The listing builds one solid part. Answer for the finished solid, in the listing's coordinates (mm). A direction names the side the tool comes from. Give positions to 0.01 mm unless a question says otherwise; leave off trailing zeros. Order: outer loops, then holes, each group sorted by start corner. A loop starts at its lowest first (then second) coordinate and runs counter-clockwise, first axis right, second up. Notation, with made-up numbers: (13.5, -17.75) - (47.5, -17.75) arc R9 ccw to (47.5, -2.75) - close; hole circle Ø5 at (-22, 0.5). An arc over 180 degrees is marked (long way). Write each question's results on one line, items separated by ' | '. Start each with the question number.
1. Section A-A (x = -12.01) is taken. Give the vertices of the cut face in (y, z), and give its area (3 significant figures).
2. Find the intervals of material crossed by L1, parallel to X at y = 18, z = -4 (3 decimals); L2, parallel to Y at x = -12.01, z = 2; L3, parallel to Y at x = 12.09, z = 2.25, in increasing order.
3. Section D-D (y = 3.8) is taken. Give the vertices of the cut face in (x, z).
4. Flat-ended cylindrical pins translate along their axes: pin 1 (2 mm diameter, centred on x = 9, z = -5.5, fed in from +Y); pin 2 (0.8 mm diameter, centred on x = -11.5, z = 6, fed in from -Y); pin 3 (6 mm diameter, centred on y = 15.5, z = 0.5, fed in from +X); pin 4 (3 mm diameter, centred on x = 11.5, y = 2, fed in from -Z). Find the tip coordinate at first contact, or state that the pin passes through.
5. Section B-B (z = 0) is taken. Give the vertices of the cut face in (x, y) (3 decimals), and give its area (3 significant figures).
6. Section C-C (x = 12.09) is taken. Give the vertices of the cut face in (y, z), and give its area (3 significant figures).
7. Determine the mould class of faces 1 (the face through (-8.464, 26.03, -0.134)), 2 (the face through (13.4, 18.4, -5.15)), 3 (the face through (13.4, 7.1, 0)), 4 (the face through (-12, 19.828, -6)) for opening direction Z: released by +Z, released by -Z, zero draft, split by the parting line, or undercut.
8. Which of the six approach directions +Z, -Z, +X, -X, +Y, -Y give full straight-line access (tool end or side, diameter ignored) to faces 5 (the face through (8.484, 26.03, 0.134)), 6 (the face through (12, 14.372, -6)), 7 (the face through (9.716, 15.755, 6.418)), 8 (the face through (11.48, 3.09, 5.38)), 9 (the face through (-13, 3, 0))?
from build123d import *

# Parameters (mm, degrees)
SKETCH1_W                    = 34.42
SKETCH1_H                    = 15.3
BOSS_EXTRUDE1_DEPTH          = 21.1
CHAMFER1_SIZE                = 3.6
CHAMFER1_SIZE2               = 2.7
CHAMFER2_SIZE                = 4.2
CHAMFER2_SIZE2               = 3.3
CUT_EXTRUDE1_DEPTH           = 32.232740834
SKETCH3_R                    = 8.475
BOSS_EXTRUDE2_DEPTH          = 10
CUT_EXTRUDE2_REACH           = 30.517
F_0_15_0_15_DIAMETER_HOLE1_D = 3.3
F_0_15_0_15_DIAMETER_HOLE2_D = 3.3
CUT_EXTRUDE3_DEPTH           = 2.5
CUT_EXTRUDE4_START           = -15.3
CUT_EXTRUDE4_DEPTH           = 2.5
SKETCH10_W                   = 6.1
SKETCH10_H                   = 6.1
CUT_EXTRUDE5_DEPTH           = 7.7
CUT_EXTRUDE6_DEPTH           = 7.7
SKETCH12_R                   = 3
BOSS_EXTRUDE3_DEPTH          = 13


with BuildPart() as part:
    # Sketch1 → Boss-Extrude1 (new body)
    with BuildSketch(Plane(origin=(0, 0, 0), x_dir=(1, 0, 0), z_dir=(0, 1, 0))):
        Rectangle(SKETCH1_W, SKETCH1_H)
    extrude(amount=BOSS_EXTRUDE1_DEPTH)

    # Chamfer1
    chamfer1_edges = [part.edges().sort_by_distance(p)[0] for p in [
        (17.21, 21.1, 0),
    ]]
    chamfer1_side = [part.faces().sort_by_distance(p)[0] for p in [
        (17.21, 10.55, 0),
    ]]
    chamfer(chamfer1_edges, length=CHAMFER1_SIZE, length2=CHAMFER1_SIZE2, reference=chamfer1_side[0])

    # Chamfer2
    chamfer2_edges = [part.edges().sort_by_distance(p)[0] for p in [
        (-17.21, 21.1, 0),
    ]]
    chamfer2_side = [part.faces().sort_by_distance(p)[0] for p in [
        (-17.21, 10.55, 0),
    ]]
    chamfer(chamfer2_edges, length=CHAMFER2_SIZE, length2=CHAMFER2_SIZE2, reference=chamfer2_side[0])

    # Sketch2 → Cut-Extrude1 (cut, through all)
    with BuildSketch(Plane.XY.offset(7.65)):
        Polygon((-17.21, 3), (-7.71, 3), (-6.91, 0), (-17.21, 0), align=None)
        Polygon((17.21, 6.1), (13.11, 6.1), (9.81, 0), (17.21, 0), align=None)
    extrude(amount=-CUT_EXTRUDE1_DEPTH, mode=Mode.SUBTRACT)

    # Sketch3 → Boss-Extrude2 (add)
    with BuildSketch(Plane(origin=(0, 21.1, 0), x_dir=(1, 0, 0), z_dir=(0, 1, 0))):
        with Locations(Location((0.01, 0, 0), (0, 0, 64.509262206))):
            Circle(SKETCH3_R)
    extrude(amount=BOSS_EXTRUDE2_DEPTH)

    # Sketch4 → Cut-Extrude2 (cut, up to next)
    with BuildSketch(Plane.XZ.offset(-21.1), mode=Mode.PRIVATE) as cut_extrude2_sk1:
        with BuildLine():
            Line((-3.637344925, -7.65), (3.657344925, -7.65))
            ThreePointArc((3.657344925, -7.65), (0.01, -8.475), (-3.637344925, -7.65))
        make_face()
    cut_extrude2_tool1 = extrude(cut_extrude2_sk1.sketch, amount=-CUT_EXTRUDE2_REACH, mode=Mode.PRIVATE) & part.part
    # Sketch4 → Cut-Extrude2 (cut, up to next)
    with BuildSketch(Plane.XZ.offset(-21.1), mode=Mode.PRIVATE) as cut_extrude2_sk2:
        with BuildLine():
            Line((-3.637344925, 7.65), (3.657344925, 7.65))
            ThreePointArc((3.657344925, 7.65), (0.01, 8.475), (-3.637344925, 7.65))
        make_face()
    cut_extrude2_tool2 = extrude(cut_extrude2_sk2.sketch, amount=-CUT_EXTRUDE2_REACH, mode=Mode.PRIVATE) & part.part
    add(cut_extrude2_tool1.solids().sort_by_distance((0.01, 21.1, -7.981417))[0], mode=Mode.SUBTRACT)
    add(cut_extrude2_tool2.solids().sort_by_distance((0.01, 21.1, 7.981417))[0], mode=Mode.SUBTRACT)

    # Ø0.15 (0.15) Diameter Hole1 (through all)
    with Locations(Plane.XY.offset(7.65)):
        with Locations((-12.01, 17.1)):
            Hole(F_0_15_0_15_DIAMETER_HOLE1_D / 2)

    # Ø0.15 (0.15) Diameter Hole2 (through all)
    with Locations(Plane.XY.offset(7.65)):
        with Locations((12.09, 17.1)):
            Hole(F_0_15_0_15_DIAMETER_HOLE2_D / 2)

    # Sketch9 → Cut-Extrude3 (cut)
    with BuildSketch(Plane.XY.offset(7.65)):
        Polygon((8.94, 17.1), (10.515, 14.372019978), (13.665, 14.372019978), (15.24, 17.1), (13.665, 19.827980022), (10.515, 19.827980022), align=None)
        Polygon((-15.16, 17.1), (-13.585, 14.372019978), (-10.435, 14.372019978), (-8.86, 17.1), (-10.435, 19.827980022), (-13.585, 19.827980022), align=None)
    extrude(amount=-CUT_EXTRUDE3_DEPTH, mode=Mode.SUBTRACT)

    # Sketch9<2> → Cut-Extrude4 (cut)
    with BuildSketch(Plane.XY.offset(7.65).offset(CUT_EXTRUDE4_START)):
        Polygon((8.94, 17.1), (10.515, 14.372019978), (13.665, 14.372019978), (15.24, 17.1), (13.665, 19.827980022), (10.515, 19.827980022), align=None)
        Polygon((-15.16, 17.1), (-13.585, 14.372019978), (-10.435, 14.372019978), (-8.86, 17.1), (-10.435, 19.827980022), (-13.585, 19.827980022), align=None)
    extrude(amount=CUT_EXTRUDE4_DEPTH, mode=Mode.SUBTRACT)

    # Sketch10 → Cut-Extrude5 (cut)
    with BuildSketch(Plane(origin=(17.21, 0, 0), x_dir=(0, 0, -1), z_dir=(1, 0, 0))):
        with Locations((0, 3.05)):
            Rectangle(SKETCH10_W, SKETCH10_H)
    extrude(amount=-CUT_EXTRUDE5_DEPTH, mode=Mode.SUBTRACT)

    # Sketch11 → Cut-Extrude6 (cut)
    with BuildSketch(Plane(origin=(17.21, 0, 0), x_dir=(0, 0, -1), z_dir=(1, 0, 0))):
        with BuildLine():
            Line((2, 6.1), (-2, 6.1))
            ThreePointArc((-2, 6.1), (0, 7.1), (2, 6.1))
        make_face()
    extrude(amount=-CUT_EXTRUDE6_DEPTH, mode=Mode.SUBTRACT)

    # Sketch12 → Boss-Extrude3 (add)
    with BuildSketch(Plane(origin=(9.51, 0, 0), x_dir=(0, 0, -1), z_dir=(1, 0, 0))):
        with Locations(Location((0, 3.8, 0), (0, 0, 180))):
            Circle(SKETCH12_R)
    extrude(amount=BOSS_EXTRUDE3_DEPTH)


solid = part.part
Reported:
1) outline: (3, -7.65) - (14.37, -7.65) - (14.37, -5.15) - (15.45, -5.15) - (15.45, 5.15) - (14.37, 5.15) - (14.37, 7.65) - (3, 7.65) - close; (18.75, -5.15) - (19.83, -5.15) - (19.83, -7.65) - (21.1, -7.65) - (21.1, 7.65) - (19.83, 7.65) - (19.83, 5.15) - (18.75, 5.15) - close | area: 216 mm²
2) L1: -16.346 to -13.393, -10.627 to 10.707, 13.473 to 16.835 | L2: 3 to 15.45, 18.75 to 21.1 | L3: 1.82 to 5.78, 6.1 to 15.45, 18.75 to 21.1
3) outline: (-17.21, -7.65) - (11.87, -7.65) - (11.87, -3.05) - (9.51, -3.05) - (9.51, -3) - (22.51, -3) - (22.51, 3) - (9.51, 3) - (9.51, 3.05) - (11.87, 3.05) - (11.87, 7.65) - (-17.21, 7.65) - close
4) pin 1: y = 21.1 | pin 2: y = 3 | pin 3: x = 17.21 | pin 4: z = -7.65
5) outline: (-17.21, 3) - (-7.71, 3) - (-6.91, 0) - (9.51, 0) - (9.51, 0.8) - (22.51, 0.8) - (22.51, 6.8) - (9.51, 6.8) - (9.51, 7.1) - (17.21, 7.1) - (17.21, 17.5) - (14.51, 21.1) - (8.485, 21.1) - (8.485, 31.1) - (-8.465, 31.1) - (-8.465, 21.1) - (-13.91, 21.1) - (-17.21, 16.9) - close; hole circle Ø3.3 at (-12.01, 17.1); hole circle Ø3.3 at (12.09, 17.1) | area: 860 mm²
6) outline: circle Ø6 at (3.8, 0); (4.21, -7.65) - (14.37, -7.65) - (14.37, -5.15) - (15.45, -5.15) - (15.45, 5.15) - (14.37, 5.15) - (14.37, 7.65) - (4.21, 7.65) - (4.21, 3.05) - (6.1, 3.05) - (6.1, 2) arc R2.5 cw to (6.1, -2) - (6.1, -3.05) - (4.21, -3.05) - close; (18.75, -5.15) - (19.83, -5.15) - (19.83, -7.65) - (21.1, -7.65) - (21.1, 7.65) - (19.83, 7.65) - (19.83, 5.15) - (18.75, 5.15) - close | area: 211 mm²
7) face 1: split by the parting line | face 2: released by -Z | face 3: undercut | face 4: zero draft
8) face 5: +X, +Y | face 6: -Z | face 7: +Z | face 8: +Z, +X, -Y | face 9: +Z, -Z, -X, -Y
